Read the model definition and answer for the solid it produces. Units are mm, in the model's axes. A direction names the side the tool comes from. Give positions to 0.01 mm unless a question says otherwise; leave off trailing zeros. Loops run counter-clockwise (first coordinate to the right, second up) from the corner with the lowest first, then second, coordinate; pieces in that order, holes last. Notation, with made-up numbers: (41.5, 16) -> (70.5, 16) arc R25 ccw to (70.5, 46) -> close; hole circle Ø11 at (-3.5, -39). An arc over 180 degrees is marked (long way). Write each question's results on one line, items separated by ' | '. Start each with the question number.
Item 1: Section C-C on x = -0.55 is taken. Write down the section's boundary in (y, z), and give its area (3 significant figures).
Item 2: Find the intervals of material crossed by line 1 (Z direction, x = 0.15, y = 0); line 2 (Y direction, x = -0.7, z = -1); line 3 (X direction, y = -1.5, z = 2.5), in increasing order.
Item 3: Section A-A on z = 0 is taken. Write down the section's boundary in (x, y).
Item 4: This flat-tipped pin is pushed along its axis until it touches: P1, Ø4, axis at y = 1.5, z = 1.5, coming from the -X side. Where does it stop, or does it pass through?
Item 5: Section D-D on z = -1.75 is taken. Write down the section's boundary in (x, y), and give its area (3 significant figures).
Item 6: Determine the mould class of faces 1 (the flat face through (1.5, 3, 1)), 2 (the flat face through (-1.3, -2, 1)), 3 (the cylindrical face through (0.021, 3.233, -1.341)) for opening direction Z: +Z half, -Z half, draft (parallel to the pull), parting line (faces both ways), or undercut.
Item 7: Which of the six approach directions +Z, -Z, +X, -X, +Y, -Y give full straight-line access (tool end or side, diameter ignored) to faces 4 (the flat face through (-1.5, 3, 1)), 5 (the flat face through (1.3, -2, -1))?
Autodesk Inventor part; units mm, degrees
ref_plane "YZ Plane" through (0, 0, 0) normal (1, 0, 0) x (0, 1, 0)
ref_plane "XZ Plane" through (0, 0, 0) normal (0, 1, 0) x (-1, 0, 0)
ref_plane "XY Plane" through (0, 0, 0) normal (0, 0, 1) x (1, 0, 0)
sketch "Sketch1" plane through (0, 0, 0) normal (1, 0, 0) x (0, 1, 0)
  circle A0 centre (0, 0) radius 1.5
  circle A1 centre (0, 0) radius 3.5
  dimension "d0" = 3
  dimension "d1" = 7
extrude "Extrusion1" add sketch "Sketch1" along normal mid plane 3
sketch "Sketch2" plane through (1.5, 0, 0) normal (1, 0, 0) x (0, 0, -1)
  circle A0 centre (0, 0) radius 2
  circle A1 centre (0, 0) radius 3
  dimension "d4" = 4
  dimension "d5" = 6
extrude "Extrusion2" cut sketch "Sketch2" against normal blind 0.2
mirror "Mirror1" about plane through (0, 0, 0) normal (1, 0, 0) of "Extrusion2"
properties part number "WheelBearings"
Findings:
1) outline: circle Ø7 at (0, 0); hole circle Ø3 at (0, 0) | area: 31.4 mm2
2) line 1: -3.5 to -1.5, 1.5 to 3.5 | line 2: -3.35 to -1.12, 1.12 to 3.35 | line 3: -1.3 to 1.3
3) outline: (-1.5, -3.5) -> (1.5, -3.5) -> (1.5, -3) -> (1.3, -3) -> (1.3, -2) -> (1.5, -2) -> (1.5, -1.5) -> (-1.5, -1.5) -> (-1.5, -2) -> (-1.3, -2) -> (-1.3, -3) -> (-1.5, -3) -> close; (-1.5, 1.5) -> (1.5, 1.5) -> (1.5, 2) -> (1.3, 2) -> (1.3, 3) -> (1.5, 3) -> (1.5, 3.5) -> (-1.5, 3.5) -> (-1.5, 3) -> (-1.3, 3) -> (-1.3, 2) -> (-1.5, 2) -> close
4) P1: x = -1.5
5) outline: (-1.5, -3.03) -> (1.5, -3.03) -> (1.5, -2.44) -> (1.3, -2.44) -> (1.3, -0.97) -> (1.5, -0.97) -> (1.5, 0.97) -> (1.3, 0.97) -> (1.3, 2.44) -> (1.5, 2.44) -> (1.5, 3.03) -> (-1.5, 3.03) -> (-1.5, 2.44) -> (-1.3, 2.44) -> (-1.3, 0.97) -> (-1.5, 0.97) -> (-1.5, -0.97) -> (-1.3, -0.97) -> (-1.3, -2.44) -> (-1.5, -2.44) -> close | area: 17.0 mm2
6) face 1: draft | face 2: undercut | face 3: parting line
7) face 4: +Z, -Z, -X, +Y, -Y | face 5: +X
